The model under review builds one solid part; all positions refer to its coordinate system, in mm. A direction names the side the tool comes from. Round coordinates to 2 decimals unless told otherwise and drop trailing zeros. Loops run counter-clockwise (first coordinate to the right, second up) from the corner with the lowest first, then second, coordinate; pieces in that order, holes last. Notation, with made-up numbers: M -27,11 L 11,11 A14 cw 11,36 Z; hole C -39.75,-26 d11. An arc over 180 degrees is marked long. Return JSON: item names as keys, results as strings. Group by question number.
Q1. Consider section B-B (y = 4.25). State the section outline as (x, z) points (3 decimals).
Q2. To check wall thickness, follow line 1 along Y through (x, z) = (-1.2, 0) (3 decimals); line 2 along Y through (x, z) = (0.4, 0); line 3 along Y through (x, z) = (1.75, -4.5). State the ranges of each line that lie inside material, in increasing order.
Q3. Consider section C-C (x = -2.5). State the section outline as (y, z) points (3 decimals).
Q4. Consider section D-D (z = -2). State the section outline as (x, y) points (1 decimal), and give its area (3 significant figures).
Q5. For faces 1 (the face through (1.565, -1.975, 4.29)), 2 (the face through (1.565, 2.728, 3.856)), 3 (the face through (1.565, 1.235, -4.541)), 4 (the face through (0, -3.12, -1.15)), list the 3-axis set-ups (+Z, -Z, +X, -X, +Y, -Y) from which the entire face can be reached by the end or side of a thin tool; tool diameter is ignored.
Q6. Clearance check with a flat-ended pin moving along its axis: pin 1 Ø1.5 at (x, z) = (-1.5, 1) entering from -Y. State where the tip first meets the part, or that it passes through.
from build123d import *

# Parameters (mm, degrees)
BASPROSKE_W         = 3.175
BASPROSKE_H         = 5.291666667
TOOTHCUT_DEPTH      = 9.129212583
TEETHCUTS_COUNT     = 18
TEETHCUTS_ANGLE     = 340
BORSKE_R            = 0.396875
BORE_DEPTH          = 50.8009144
SKETCH1_R           = 2.778125
CUT_EXTRUDE2_DEPTH  = 1.5875
SKETCH3_R           = 3.175
SKETCH3_R_2         = 0.396875
BOSS_EXTRUDE1_DEPTH = 3.175
SKETCH4_R           = 2.38125
CUT_EXTRUDE3_DEPTH  = 4.7625


with BuildPart() as part:
    # BasProSke → Base-Revolve (revolve)
    with BuildSketch(Plane(origin=(0, 0, 0), x_dir=(1, 0, 0), z_dir=(0, 1, 0)), mode=Mode.PRIVATE) as base_revolve_sk:
        with Locations((1.5875, 2.645833334)):
            Rectangle(BASPROSKE_W, BASPROSKE_H)
    revolve(base_revolve_sk.sketch.rotate(Axis((-10, 0, 0), (1, 0, 0)), 180), axis=Axis((-10, 0, 0), (1, 0, 0)))

    # TooCutSke → ToothCut (cut, through all)
    with BuildSketch(Plane(origin=(0, 0, 0), x_dir=(0, 0, -1), z_dir=(1, 0, 0))):
        with BuildLine():
            ThreePointArc((0.270003318, 4.067748898), (0, 4.0767), (-0.270003318, 4.067748898))
            ThreePointArc((-0.270003318, 4.067748898), (-0.437425956, 4.709129954), (-0.814487039, 5.254313352))
            ThreePointArc((-0.814487039, 5.254313352), (0, 5.317066667), (0.814487039, 5.254313352))
            ThreePointArc((0.814487039, 5.254313352), (0.437425956, 4.709129954), (0.270003318, 4.067748898))
        make_face()
    toothcut = extrude(amount=TOOTHCUT_DEPTH, mode=Mode.SUBTRACT)

    # TeethCuts: ToothCut ×18 about axis
    teethcuts_axis = Axis((-10, 0, 0), (1, 0, 0))
    for i in range(1, TEETHCUTS_COUNT):
        add(toothcut.rotate(teethcuts_axis, i * TEETHCUTS_ANGLE / (TEETHCUTS_COUNT - 1)), mode=Mode.SUBTRACT)

    # BorSke → Bore (cut, symmetric)
    with BuildSketch(Plane(origin=(0, 0, 0), x_dir=(0, 0, -1), z_dir=(1, 0, 0))):
        with Locations(Location((0, 0, 0), (0, 0, 180))):
            Circle(BORSKE_R)
    extrude(amount=BORE_DEPTH, both=True, mode=Mode.SUBTRACT)

    # Sketch1 → Cut-Extrude2 (cut)
    with BuildSketch(Plane.ZY):
        Circle(SKETCH1_R)
    extrude(amount=-CUT_EXTRUDE2_DEPTH, mode=Mode.SUBTRACT)

    # Sketch3 → Boss-Extrude1 (add)
    with BuildSketch(Plane.ZY):
        with Locations(Location((0, 0, 0), (0, 0, 180))):
            Circle(SKETCH3_R)
        Circle(SKETCH3_R_2, mode=Mode.SUBTRACT)
    extrude(amount=BOSS_EXTRUDE1_DEPTH)

    # Sketch4 → Cut-Extrude3 (cut)
    with BuildSketch(Plane(origin=(3.175, 0, 0), x_dir=(0, 0, -1), z_dir=(1, 0, 0))):
        with Locations(Location((0, 0, 0), (0, 0, 180))):
            Circle(SKETCH4_R)
    extrude(amount=-CUT_EXTRUDE3_DEPTH, mode=Mode.SUBTRACT)


solid = part.part
Values:
{
 "1": {"outline": "M 0,-2.754 L 3.175,-2.754 L 3.175,-1.997 L 0,-1.997 Z; M 0,-1.198 L 3.175,-1.198 L 3.175,-0.294 L 0,-0.294 Z; M 0,0.294 L 3.175,0.294 L 3.175,1.198 L 0,1.198 Z; M 0,1.997 L 3.175,1.997 L 3.175,2.754 L 0,2.754 Z"},
 "2": {"line 1": "y = -3.175 to -2.381, 2.381 to 3.175", "line 2": "y = -4.08 to -2.78, 2.78 to 4.08", "line 3": "y = -1.98 to -1.21, -0.43 to 0.43, 1.21 to 1.98"},
 "3": {"outline": "C 0,0 d6.35; hole C 0,0 d0.794"},
 "4": {"outline": "M -3.2,-2.5 L 0,-2.5 L 0,-4.3 L 3.2,-4.3 L 3.2,-1.3 L 1.6,-1.3 L 1.6,-1.9 L 0,-1.9 L 0,-1.3 L -1.6,-1.3 L -1.6,1.3 L 0,1.3 L 0,1.9 L 1.6,1.9 L 1.6,1.3 L 3.2,1.3 L 3.2,4.3 L 0,4.3 L 0,2.5 L -3.2,2.5 Z", "area": "28.3 mm2"},
 "5": {"face 1": "+X, -X", "face 2": "+Z, +X, -X", "face 3": "-Z, +X, -X", "face 4": "-X"},
 "6": {"pin 1": "stops at y = -3.17"}
}
